CAD build for the part. Positions are in the model's coordinates, mm. A direction names the side the tool comes from. Coordinates: 2 decimals unless noted, no trailing zeros. Write each loop counter-clockwise with the first axis right and the second up, starting at its lowest first coordinate (ties: lowest second). Pieces come first, ordered by that corner, then holes. Notation, with made-up numbers: (-33, -34.75) - (-29, -34.75) arc R30 cw to (-29, -9.75) - close; hole circle Ø4 at (-14.75, 78). An arc over 180 degrees is marked (long way). Answer in a Markdown table with one row per item. Add a question column.
Q1. Pin check, flat tips, straight feed: pin 1 (2 mm diameter, centred on x = -3, z = 43.5, fed in from -Y); pin 2 (1 mm diameter, centred on y = 3.5, z = 16.5, fed in from +X); pin 3 (4 mm diameter, centred on y = 6.5, z = 54.5, fed in from -X). Stop position of each tip, or through.
Q2. Drill centre lines: line 1 along Y through (x, z) = (-6, 74); line 2 along Z through (x, y) = (-9, -0.25); line 3 along X through (y, z) = (-0.5, 47). Where is each one in solid material? Low to high. Write a range as from..to.
Q3. 3-axis set-ups, long thin cutter, end or side, ignore diameter. For faces 1 (the flat face through (-4.5, 7.4, 95)), 2 (the flat face through (0, 0, 0)): which of +Z, -Z, +X, -X, +Y, -Y reach the whole face in a straight line?
Q4. Band-saw the part on A-A (z = 105). List the corners of the cut face in (x, y), and give its area (3 significant figures).
```python
from build123d import *

# Parameters (mm, degrees)
SZKIC1_R                    = 10
DODANIE_WYCI_GNI_CIE1_DEPTH = 155
SFAZOWANIE2_SIZE            = 2
SZKIC2_W                    = 1.5
SZKIC2_H                    = 1.2


with BuildPart() as part:
    # Szkic1 → Dodanie-wyciągnięcie1 (new body)
    with BuildSketch(Plane.XY):
        Circle(SZKIC1_R)
    extrude(amount=DODANIE_WYCI_GNI_CIE1_DEPTH)

    # Sfazowanie2
    sfazowanie2_edges = [part.edges().sort_by_distance(p)[0] for p in [
        (-10, 0, 155),
    ]]
    chamfer(sfazowanie2_edges, length=SFAZOWANIE2_SIZE)

    # Szkic2 → Wycięcie-obrót1 (revolve, cut)
    with BuildSketch(Plane(origin=(0, 0, 0), x_dir=(1, 0, 0), z_dir=(0, 1, 0)), mode=Mode.PRIVATE) as wyci_cie_obr_t1_sk:
        with Locations((9.25, -94.4)):
            Rectangle(SZKIC2_W, SZKIC2_H)
    revolve(wyci_cie_obr_t1_sk.sketch.rotate(Axis((0, 0, 0), (0, 0, 1)), 180), axis=Axis((0, 0, 0), (0, 0, 1)), mode=Mode.SUBTRACT)


solid = part.part
```
Checked values:
| question | item | result |
|---|---|---|
| 1 | pin 1 | stops at y = -9.8 |
| 1 | pin 2 | stops at x = 9.54 |
| 1 | pin 3 | stops at x = -8.93 |
| 2 | line 1 | y = -8..8 |
| 2 | line 2 | z = 0..93.8, 95..154 |
| 2 | line 3 | x = -9.99..9.99 |
| 3 | face 1 | none |
| 3 | face 2 | -Z, +X, -X, +Y, -Y |
| 4 | outline | circle Ø20 at (0, 0) |
| 4 | area | 314 mm² |
